Source: three-view drawing plus pictorial views. Frame: mm from the lowest corner of the part. A direction names the side the tool comes from. Give positions to 0.01 mm unless a question says otherwise; leave off trailing zeros. Order: outer loops, then holes, each group sorted by start corner. A loop starts at its lowest first (then second) coordinate and runs counter-clockwise, first axis right, second up. Notation, with made-up numbers: (72.25, 77.25) - (95.25, 77.25) arc R11 ccw to (95.25, 91.25) - close; hole circle Ø3 at (59, 40). An arc over 180 degrees is marked (long way). Use CSV: the item, a comma, the result in double quotes.
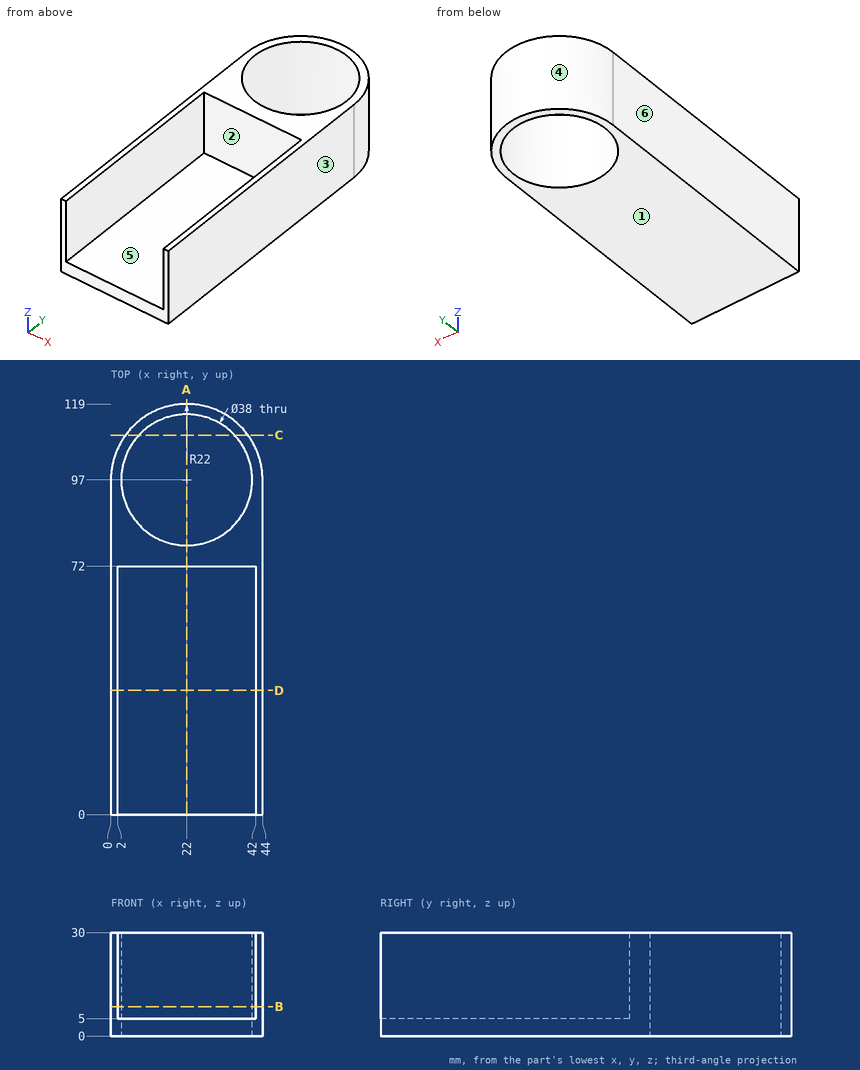
Item 1: Section A-A on x = 22. Return the cut outline in (y, z).
Filled in:
outline,"(0, 0) - (78, 0) - (78, 30) - (72, 30) - (72, 5) - (0, 5) - close; (116, 0) - (119, 0) - (119, 30) - (116, 30) - close"
Item 2: Section D-D on y = 36. Return the cut outline in (x, z).
Filled in:
outline,"(0, 0) - (44, 0) - (44, 30) - (42, 30) - (42, 5) - (2, 5) - (2, 30) - (0, 30) - close"
Item 3: Set-up query: the marked faces 5 and 6. Return all of +Z, -Z, +X, -X, +Y, -Y with unobstructed straight access to the full face (end or side cutting, diameter ignored); none if empty.
Filled in:
face 5,"+Z, -Y"
face 6,"+Z, -Z, -X, +Y, -Y"
Item 4: Section C-C on y = 110. Return the cut outline in (x, z).
Filled in:
outline,"(4.25, 0) - (8.14, 0) - (8.14, 30) - (4.25, 30) - close; (35.86, 0) - (39.75, 0) - (39.75, 30) - (35.86, 30) - close"
Item 5: First-contact query: pin 1 (3 mm diameter, centred on x = 19.5, z = 22, fed in from +Y); pin 2 (6 mm diameter, centred on x = 24.5, z = 13.5, fed in from -Y); pin 3 (1.5 mm diameter, centred on x = 38.5, y = 54.5, fed in from -Z). Flat tips, straight axial feed; report the tip coordinate or a pass-through.
Filled in:
pin 1,"stops at y = 118.98"
pin 2,"stops at y = 72"
pin 3,"stops at z = 0"
Item 6: Section B-B on z = 8.5. Return the cut outline in (x, y), then the cut area to 3 significant figures.
Filled in:
outline,"(0, 0) - (2, 0) - (2, 72) - (42, 72) - (42, 0) - (44, 0) - (44, 97) arc R22 ccw to (0, 97) - close; hole circle Ø38 at (22, 97)"
area,"1,010 mm2"
Item 7: Mould query, pull axis X, two halves, no side actions, for the marked faces 1, 2, 3 and 4. Classes: released by +X, released by -X, zero draft, split by the parting line, or undercut.
Filled in:
face 1,"zero draft"
face 2,"undercut"
face 3,"released by +X"
face 4,"split by the parting line"
Item 8: Material intervals for line 1 (Y direction, x = 22, z = 6); line 2 (X direction, y = 38, z = 10.25); line 3 (Y direction, x = 16.5, z = 18.75), sorted ascending. Write a range as from..to.
Filled in:
line 1,"y = 72..78, 116..119"
line 2,"x = 0..2, 42..44"
line 3,"y = 72..78.81, 115.19..118.3"
